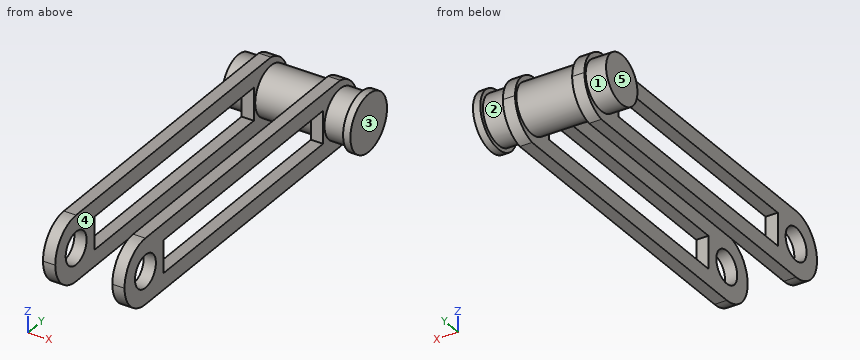
from build123d import *

# Parameters (mm, degrees)
F0_R          = 30
F1_DEPTH      = 160
F2_W          = 100
F2_H          = 80
F3_DEPTH      = 32.5
F3_DEPTH_BACK = 32.5
F4_W          = 15
F4_H          = 20
F5_DEPTH      = 380
F6_W          = 75
F6_H          = 80
F7_DEPTH      = 15
F8_W          = 75
F8_H          = 80
F9_DEPTH      = 15
F10_R         = 20
F11_DEPTH     = 135.001
F13_DEPTH     = 125.001
F14_W         = 70
F14_H         = 80
F15_DEPTH     = 65.001
F17_DEPTH     = 125.001
F18_R         = 30
F19_DEPTH     = 70
F20_R         = 35
F21_DEPTH     = 9


with BuildPart() as f1:
    # F0 (on Right) → F1 (new body)
    with BuildSketch(Plane.YZ):
        Circle(F0_R)
    extrude(amount=F1_DEPTH)

    # F2 (on Front) → F3 (join, two sides)
    with BuildSketch(Plane.XZ) as f3_sk:
        with Locations((75, 0)):
            Rectangle(F2_W, F2_H)
    extrude(amount=F3_DEPTH)
    extrude(f3_sk.sketch, amount=-F3_DEPTH_BACK)

    # F4 (on face) → F5 (join)
    with BuildSketch(Plane.XZ.offset(32.5)):
        with Locations((117.5, 30)):
            Rectangle(F4_W, F4_H)
        with Locations((117.5, -30)):
            Rectangle(F4_W, F4_H)
        with Locations((32.5, 30)):
            Rectangle(F4_W, F4_H)
        with Locations((32.5, -30)):
            Rectangle(F4_W, F4_H)
    extrude(amount=F5_DEPTH)

    # F6 (on face) → F7 (join)
    with BuildSketch(Plane.YZ.offset(125)):
        with Locations((-375, 0)):
            Rectangle(F6_W, F6_H)
    extrude(amount=-F7_DEPTH)

    # F8 (on face) → F9 (join)
    with BuildSketch(Plane(origin=(25, 0, 0), x_dir=(0, -1, 0), z_dir=(-1, 0, 0))):
        with Locations((375, 0)):
            Rectangle(F8_W, F8_H)
    extrude(amount=-F9_DEPTH)

    # F10 (on face) → F11 (cut, through all)
    with BuildSketch(Plane(origin=(25, 0, 0), x_dir=(0, -1, 0), z_dir=(-1, 0, 0))):
        with Locations((372.5, 0)):
            Circle(F10_R)
    extrude(amount=-F11_DEPTH, mode=Mode.SUBTRACT)

    # F12 (on face) → F13 (cut, through all)
    with BuildSketch(Plane.YZ.offset(125)):
        with BuildLine():
            ThreePointArc((-372.5, -40), (-400.7842712969, -28.2842711981), (-412.5, 1.397e-07))
            Line((-412.5, 1.397e-07), (-412.5, -40))
            Line((-412.5, -40), (-372.5, -40))
        make_face()
        with BuildLine():
            ThreePointArc((-412.5, 1.397e-07), (-400.7842711981, 28.2842712969), (-372.5, 40))
            Line((-372.5, 40), (-412.5, 40))
            Line((-412.5, 40), (-412.5, 1.397e-07))
        make_face()
    extrude(amount=-F13_DEPTH, mode=Mode.SUBTRACT)

    # F14 (on face) → F15 (cut, through all)
    with BuildSketch(Plane.XZ.offset(32.5)):
        with Locations((75, 0)):
            Rectangle(F14_W, F14_H)
    extrude(amount=-F15_DEPTH, mode=Mode.SUBTRACT)

    # F16 (on face) → F17 (cut, through all)
    with BuildSketch(Plane.YZ.offset(125)):
        with BuildLine():
            ThreePointArc((0, 40), (23.3508126253, 25.7694100117), (32.5, -3.825e-07))
            Line((32.5, -3.825e-07), (32.5, 40))
            Line((32.5, 40), (0, 40))
        make_face()
        with BuildLine():
            ThreePointArc((32.5, -3.825e-07), (23.3508123842, -25.7694103085), (0, -40))
            Line((0, -40), (32.5, -40))
            Line((32.5, -40), (32.5, -3.825e-07))
        make_face()
    extrude(amount=-F17_DEPTH, mode=Mode.SUBTRACT)

    # F18 (on face) → F19 (join)
    with BuildSketch(Plane(origin=(110, 0, 0), x_dir=(0, -1, 0), z_dir=(-1, 0, 0))):
        Circle(F18_R)
    extrude(amount=F19_DEPTH)

    # F20 (on face) → F21 (join)
    with BuildSketch(Plane.YZ.offset(160)):
        Circle(F20_R)
    extrude(amount=-F21_DEPTH)


solid = f1.part
Work out the finished part from the listing and answer in its coordinate system (mm). Face numbers are marked on the shaded views. A direction names the side the tool comes from. Round coordinates to 2 decimals unless told otherwise and drop trailing zeros. Loops run counter-clockwise (first coordinate to the right, second up) from the corner with the lowest first, then second, coordinate; pieces in that order, holes last. Notation, with made-up numbers: (33.5, 80) - (87.5, 80) arc R30 ccw to (87.5, 103) - close; hole circle Ø7 at (36.25, -38.5). An arc over 180 degrees is marked (long way). Use one line per item in the form item = value. Start each with the question number.
(1) Find section B-B on z = -10.5. Give the number of separate pieces and of enclosed holes in the cut face, and give its area (3 significant figures).
(2) Determine the mould class of the marked faces 3, 4 and 5 for opening direction X: +X half, -X half, draft (parallel to the pull), parting line (faces both ways), or undercut.
(3) Find section C-C on x = 146.5. Determine the outline of the cut face in (y, z), and give its area (3 significant figures).
(4) Find section A-A on y = -111. Determine the outline of the cut face in (x, z), and give its area (3 significant figures).
(5) Which of the six approach directions +Z, -Z, +X, -X, +Y, -Y give full straight-line access (tool end or side, diameter ignored) to the marked faces 1 and 2?
(6) Flat-ended cylindrical pins translate along their axes: P1, Ø5, axis at x = 104, z = -29.5, coming from the -Y side; P2, Ø3, axis at x = 39.5, z = -27.5, coming from the +Y side; P3, Ø7.5, axis at x = 121, z = 10, coming from the +Y side. Find the tip coordinate at first contact, or state that the pin passes through.
(7) Consider line 1 (Z direction, x = 120, y = -372.5); line 2 (X direction, y = -213.5, z = -32); line 3 (Y direction, x = 107, z = 1). Determine where each line is inside the solid, lowest interval first.
Answer list:
q1.separate_pieces = 5
q1.enclosed_holes = 0
q1.area = 10,500 mm^2
q2.face_3 = +X half
q2.face_4 = undercut
q2.face_5 = -X half
q3.outline = circle Ø60 at (0, 0)
q3.area = 2,830 mm^2
q4.outline = (25, -40) - (40, -40) - (40, -20) - (25, -20) - close; (25, 20) - (40, 20) - (40, 40) - (25, 40) - close; (110, -40) - (125, -40) - (125, -20) - (110, -20) - close; (110, 20) - (125, 20) - (125, 40) - (110, 40) - close
q4.area = 1,200 mm^2
q5.face_1 = -X
q5.face_2 = none
q6.P1 = -13.08
q6.P2 = 23.16
q6.P3 = 32.02
q7.line_1 = -40 to -20, 20 to 40
q7.line_2 = 25 to 40, 110 to 125
q7.line_3 = -29.98 to 29.98
